```python
from build123d import *

# Parameters (mm, degrees)
SKETCH1_R                            = 12.2555
SKETCH1_R_2                          = 10.9855
BOSS_EXTRUDE1_DEPTH                  = 25.4
CUT_EXTRUDE1_DEPTH                   = 31.749870902
CUT_EXTRUDE1_DEPTH_BACK              = 31.749870902
SKETCH2_W                            = 7.874
SKETCH2_H                            = 0.935
SKETCH8_W                            = 25.4
SKETCH8_H                            = 6.35
BOSS_EXTRUDE2_DEPTH                  = 11.43
BOSS_EXTRUDE2_DIRECTION_2_REACH      = 39.365
BOSS_EXTRUDE2_DIRECTION_2_END_RADIUS = 12.2555
SKETCH9_R                            = 1.4605
CUT_EXTRUDE6_DEPTH                   = 39.003463533
SKETCH10_W                           = 3.175
SKETCH10_H                           = 7.62
CUT_EXTRUDE7_DEPTH                   = 25.4
FILLET2_R                            = 2.54
SKETCH11_R                           = 10.9855
CUT_EXTRUDE8_DEPTH                   = 37.82879567
SKETCH12_R                           = 1.2875
BOSS_EXTRUDE3_DEPTH                  = 2.196999908
BOSS_EXTRUDE4_START                  = -25.4
BOSS_EXTRUDE4_DEPTH                  = 25.4
FILLET3_R                            = 5.08
FILLET3_OF_MIRROR2_R                 = 5.08
CUT_EXTRUDE9_DEPTH                   = 43.697648058
CUT_EXTRUDE9_DEPTH_BACK              = 43.697648058
SKETCH13_W                           = 17.526
SKETCH13_H                           = 2.120056883
SKETCH13_W_2                         = 0.599999908
SKETCH13_H_2                         = 18.990443025
FILLET4_R                            = 5.08
CUT_EXTRUDE10_DEPTH                  = 37.861439453
CUT_EXTRUDE10_DEPTH_BACK             = 37.861439453
SKETCH17_W                           = 24.800000092
SKETCH17_H                           = 8.799318797
CUT_EXTRUDE11_DEPTH                  = 2.54
CUT_EXTRUDE11_DEPTH_BACK             = 37.940724096
SKETCH18_W                           = 7.62
SKETCH18_H                           = 1.148317315
SKETCH18_H_2                         = 1.391682685
CUT_EXTRUDE12_DEPTH                  = 36.881723087
CUT_EXTRUDE12_DEPTH_BACK             = 36.881723087
SKETCH19_W                           = 6.050000046
SKETCH19_H                           = 17.461181295


with BuildPart() as part:
    # Sketch1 → Boss-Extrude1 (new body)
    with BuildSketch(Plane(origin=(0, 0, 0), x_dir=(0, 0, -1), z_dir=(1, 0, 0))):
        Circle(SKETCH1_R)
        Circle(SKETCH1_R_2, mode=Mode.SUBTRACT)
    extrude(amount=BOSS_EXTRUDE1_DEPTH)

    # Sketch2 → Cut-Extrude1 (cut, two sides: drawn at the far end of the back side and taken through both)
    with BuildSketch(Plane(origin=(0, 0, 0), x_dir=(1, 0, 0), z_dir=(0, 1, 0)).offset(-CUT_EXTRUDE1_DEPTH_BACK)):
        with Locations((21.463, 11.788)):
            Rectangle(SKETCH2_W, SKETCH2_H)
        with Locations((21.463, -11.788)):
            Rectangle(SKETCH2_W, SKETCH2_H)
    extrude(amount=CUT_EXTRUDE1_DEPTH + CUT_EXTRUDE1_DEPTH_BACK, mode=Mode.SUBTRACT)

    # Sketch8 → Boss-Extrude2 (add)
    with BuildSketch(Plane(origin=(0, 12.2555, 0), x_dir=(1, 0, 0), z_dir=(0, 1, 0))):
        with Locations((12.7, 0)):
            Rectangle(SKETCH8_W, SKETCH8_H)
    extrude(amount=BOSS_EXTRUDE2_DEPTH)

    # Boss-Extrude2 direction 2: up to this cylinder (the profile starts outside it)
    boss_extrude2_direction_2_end = Plane(origin=(12.7, 0, 0), z_dir=(-1, 0, 0)) * Cylinder(BOSS_EXTRUDE2_DIRECTION_2_END_RADIUS, 104.241, mode=Mode.PRIVATE)
    # Sketch8 → Boss-Extrude2 direction 2 (add, up to the surface)
    with BuildSketch(Plane(origin=(0, 12.2555, 0), x_dir=(1, 0, 0), z_dir=(0, 1, 0)), mode=Mode.PRIVATE) as boss_extrude2_direction_2_sk1:
        with Locations((12.7, 0)):
            Rectangle(SKETCH8_W, SKETCH8_H)
    boss_extrude2_direction_2_tool1 = extrude(boss_extrude2_direction_2_sk1.sketch, amount=-BOSS_EXTRUDE2_DIRECTION_2_REACH, mode=Mode.PRIVATE) - boss_extrude2_direction_2_end
    add(boss_extrude2_direction_2_tool1.solids().sort_by_distance((12.7, 12.2555, 0))[0])
    add(boss_extrude2_direction_2_tool1.solids().sort_by_distance((12.7, 12.2555, 0))[1])

    # Sketch9 → Cut-Extrude6 (cut, through all)
    with BuildSketch(Plane(origin=(0, 0, -3.175), x_dir=(-1, 0, 0), z_dir=(0, 0, -1))):
        with Locations((-12.7, 19.685)):
            Circle(SKETCH9_R)
    extrude(amount=-CUT_EXTRUDE6_DEPTH, mode=Mode.SUBTRACT)

    # Sketch10 → Cut-Extrude7 (cut)
    with BuildSketch(Plane.ZY):
        with Locations((0, 19.8755)):
            Rectangle(SKETCH10_W, SKETCH10_H)
    extrude(amount=-CUT_EXTRUDE7_DEPTH, mode=Mode.SUBTRACT)

    # Fillet2
    fillet2_edges = [part.edges().sort_by_distance(p)[0] for p in [
        (12.7, 11.837088124, 3.175),
        (12.7, 11.837088124, -3.175),
    ]]
    fillet(fillet2_edges, radius=FILLET2_R)

    # Sketch11 → Cut-Extrude8 (cut, through all)
    with BuildSketch(Plane(origin=(25.4, 0, 0), x_dir=(0, 0, -1), z_dir=(1, 0, 0))):
        with BuildLine():
            ThreePointArc((-10.9855, 0), (-10.718799827, -2.405938595), (-9.931648919, -4.695056975))
            Line((-9.931648919, -4.695056975), (9.931648919, -4.695056975))
            ThreePointArc((9.931648919, -4.695056975), (10.718799827, -2.405938595), (10.9855, 0))
            Line((10.9855, 0), (-10.9855, 0))
        make_face()
        with BuildLine():
            Line((9.931648919, -4.695056975), (-9.931648919, -4.695056975))
            ThreePointArc((-9.931648919, -4.695056975), (0, -10.9855), (9.931648919, -4.695056975))
        make_face()
        Circle(SKETCH11_R)
        with BuildLine():
            Line((-11.3205, -4.695056975), (11.3205, -4.695056975))
            ThreePointArc((11.3205, -4.695056975), (0, -12.2555), (-11.3205, -4.695056975))
        make_face()
        with BuildLine():
            Line((-11.3205, -4.695056975), (-11.3205, -12.703036631))
            Line((-11.3205, -12.703036631), (11.3205, -12.703036631))
            Line((11.3205, -12.703036631), (11.3205, -4.695056975))
            ThreePointArc((11.3205, -4.695056975), (0, -12.2555), (-11.3205, -4.695056975))
        make_face()
        with BuildLine():
            Line((-10.9855, 0), (-10.9855, -4.695056975))
            Line((-10.9855, -4.695056975), (-9.931648919, -4.695056975))
            ThreePointArc((-9.931648919, -4.695056975), (-10.718799827, -2.405938595), (-10.9855, 0))
        make_face()
        with BuildLine():
            Line((9.931648919, -4.695056975), (10.9855, -4.695056975))
            Line((10.9855, -4.695056975), (10.9855, 0))
            ThreePointArc((10.9855, 0), (10.718799827, -2.405938595), (9.931648919, -4.695056975))
        make_face()
    extrude(amount=-CUT_EXTRUDE8_DEPTH, mode=Mode.SUBTRACT)

    # Sketch12 → Boss-Extrude3 (add)
    with BuildSketch(Plane(origin=(0, 0, -11.3205), x_dir=(-1, 0, 0), z_dir=(0, 0, -1))):
        with Locations(Location((-22.225, 0, 0), (0, 0, 180))):
            Circle(SKETCH12_R)
    boss_extrude3 = extrude(amount=BOSS_EXTRUDE3_DEPTH)

    # Mirror1: Boss-Extrude3 across plane
    add(boss_extrude3.mirror(Plane.XY))

    # Sketch14 → Boss-Extrude4 (add)
    with BuildSketch(Plane(origin=(25.4, 0, 0), x_dir=(0, 0, -1), z_dir=(1, 0, 0)).offset(BOSS_EXTRUDE4_START)):
        with BuildLine():
            ThreePointArc((-9.8205, 4.923310878), (-10.690283275, 2.529635102), (-10.9855, 0))
            Line((-10.9855, 0), (-10.9855, -4.695056975))
            Line((-10.9855, -4.695056975), (-9.8205, -4.695056975))
            Line((-9.8205, -4.695056975), (-9.8205, 4.923310878))
        make_face()
    boss_extrude4 = extrude(amount=BOSS_EXTRUDE4_DEPTH)

    # Fillet3
    fillet3_edges = [part.edges().sort_by_distance(p)[0] for p in [
        (12.7, 4.923310878, 9.8205),
    ]]
    fillet(fillet3_edges, radius=FILLET3_R)

    # Mirror2: Boss-Extrude4 across plane
    add(boss_extrude4.mirror(Plane.XY))

    # Fillet3 of Mirror2
    fillet3_of_mirror2_edges = [part.edges().sort_by_distance(p)[0] for p in [
        (12.7, 4.923310878, -9.8205),
    ]]
    fillet(fillet3_of_mirror2_edges, radius=FILLET3_OF_MIRROR2_R)

    # Sketch13 → Cut-Extrude9 (cut, two sides: drawn at the far end of the back side and taken through both)
    with BuildSketch(Plane(origin=(0, 0, -11.3205), x_dir=(-1, 0, 0), z_dir=(0, 0, -1)).offset(-CUT_EXTRUDE9_DEPTH_BACK)):
        with BuildLine():
            ThreePointArc((-22.225, -2.575000092), (-24.045800027, -1.820800027), (-24.800000092, 0))
            Line((-24.800000092, 0), (-24.800000092, 4.695056975))
            Line((-24.800000092, 4.695056975), (-25.4, 4.695056975))
            Line((-25.4, 4.695056975), (-25.4, -4.695056975))
            Line((-25.4, -4.695056975), (-17.526, -4.695056975))
            Line((-17.526, -4.695056975), (-17.526, -2.575000092))
            Line((-17.526, -2.575000092), (-22.225, -2.575000092))
        make_face()
        with Locations((-8.763, -3.635028533)):
            Rectangle(SKETCH13_W, SKETCH13_H)
        with Locations((-25.100000046, 14.190278488)):
            Rectangle(SKETCH13_W_2, SKETCH13_H_2)
    extrude(amount=CUT_EXTRUDE9_DEPTH + CUT_EXTRUDE9_DEPTH_BACK, mode=Mode.SUBTRACT)

    # Fillet4
    fillet4_edges = [part.edges().sort_by_distance(p)[0] for p in [
        (24.800000092, 23.6855, -2.38125),
        (24.800000092, 23.6855, 2.38125),
        (0, 23.6855, -2.38125),
        (0, 23.6855, 2.38125),
    ]]
    fillet(fillet4_edges, radius=FILLET4_R)

    # Sketch17 → Cut-Extrude10 (cut, two sides: drawn at the far end of the back side and taken through both)
    with BuildSketch(Plane.XY.offset(-CUT_EXTRUDE10_DEPTH_BACK)):
        with Locations((12.400000046, 1.824659306)):
            Rectangle(SKETCH17_W, SKETCH17_H)
    extrude(amount=CUT_EXTRUDE10_DEPTH + CUT_EXTRUDE10_DEPTH_BACK, mode=Mode.SUBTRACT)

    # Sketch18 → Cut-Extrude11 (cut, two sides: drawn at the far end of the back side and taken through both)
    with BuildSketch(Plane(origin=(0, 0, -3.175), x_dir=(-1, 0, 0), z_dir=(0, 0, -1)).offset(-CUT_EXTRUDE11_DEPTH_BACK)):
        with Locations((-12.400000046, 14.221341343)):
            Rectangle(SKETCH18_W, SKETCH18_H)
        with Locations((-12.400000046, 12.951341343)):
            Rectangle(SKETCH18_W, SKETCH18_H_2)
    extrude(amount=CUT_EXTRUDE11_DEPTH + CUT_EXTRUDE11_DEPTH_BACK, mode=Mode.SUBTRACT)

    # Sketch19 → Cut-Extrude12 (cut, two sides: drawn at the far end of the back side and taken through both)
    with BuildSketch(Plane.XY.offset(-CUT_EXTRUDE12_DEPTH_BACK)):
        with Locations((3.025000023, 14.954909352)):
            Rectangle(SKETCH19_W, SKETCH19_H)
        with Locations((21.775000069, 14.954909352)):
            Rectangle(SKETCH19_W, SKETCH19_H)
    extrude(amount=CUT_EXTRUDE12_DEPTH + CUT_EXTRUDE12_DEPTH_BACK, mode=Mode.SUBTRACT)


solid = part.part
```
The model under review builds one solid part; all positions refer to its coordinate system, in mm. A direction names the side the tool comes from. Round coordinates to 2 decimals unless told otherwise and drop trailing zeros. Loops run counter-clockwise (first coordinate to the right, second up) from the corner with the lowest first, then second, coordinate; pieces in that order, holes last. Notation, with made-up numbers: M 25,8 L 38,8 A9 cw 38,14 Z; hole C 0,-17 d6. An arc over 180 degrees is marked long. Put each result on its own line as item: value.
Q1. Mouldability with a two-part tool opening along Z and no side actions: class faces 5 (the cylindrical face through (12.31, 11.99, -3.79)), 6 (the cylindrical face through (12.311, 10.985, -0.143)), 7 (the flat face through (12, 6.224, -10)) as released by +Z, released by -Z, zero draft, split by the parting line, or undercut.
Result set:
face 5: released by -Z
face 6: undercut
face 7: zero draft
Q2. Machinability: for faces 1 (the flat face through (11, 20, 1.588)), 2 (the flat face through (12, 12.256, 0)), 3 (the flat face through (12, 18, 3.175)), 4 (the flat face through (12, 6.224, 10)), which of the approach directions +Z, -Z, +X, -X, +Y, -Y give a long, thin tool a straight path to every point of the face, cutting with its end or side? Answer none if there is none.
Result set:
face 1: +X, -X, +Y
face 2: +Z, -Z
face 3: +Z, +X, -X, +Y
face 4: +Z, -Z, +X, -X, -Y
Q3. Consider section A-A, the plane x = 12.7. Count the separate pieces of the cut face and the enclosed holes in it, then the cut area to 3 significant figures.
Result set:
separate pieces: 4
enclosed holes: 0
area: 54.3 mm²
Q4. Consider section C-C, the plane z = 0. Give the boundary of the cut face in (x, y).
Result set:
outline: M 6.05,10.99 L 18.75,10.99 L 18.75,16.07 L 6.05,16.07 Z; hole M 8.59,12.26 L 16.21,12.26 L 16.21,14.8 L 8.59,14.8 Z
Q5. To check wall thickness, follow L1, parallel to Y at x = 12.7, z = -2; L2, parallel to Y at x = 12.7, z = -2.6; L3, parallel to X at y = 14, z = -0.25. State the ranges of each line that lie inside material, in increasing order.
Result set:
L1: y = 10.8 to 12.26, 14.8 to 18.22, 21.15 to 23.69
L2: y = 10.67 to 12.26, 14.8 to 18.22, 21.15 to 23.69
L3: x = 6.05 to 8.59, 16.21 to 18.75
Q6. For pin 1 (5 mm diameter, centred on x = 10.5, y = 17.5, fed in from -Z) (3 decimals); pin 2 (5 mm diameter, centred on x = 13.5, z = 1, fed in from -Y); pin 3 (2.5 mm diameter, centred on x = 9.5, y = 21, fed in from +Z) (3 decimals), all flat-tipped, find the tip position at first contact; note any pin that passes through.
Result set:
pin 1: stops at z = -3.175
pin 2: stops at y = 10.41
pin 3: stops at z = 3.175
